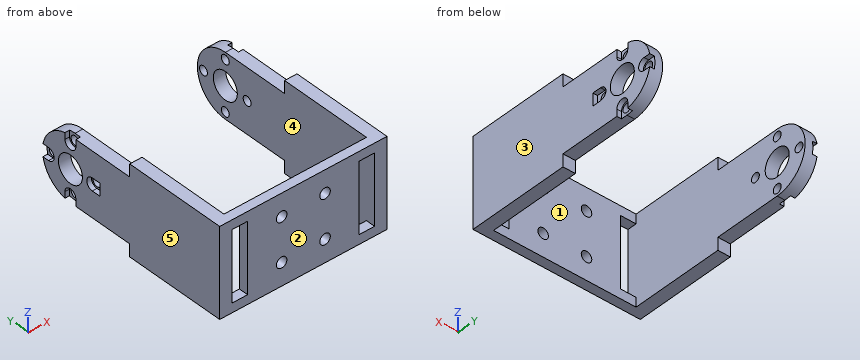
```python
from build123d import *
from build123d.topology import SkipClean

# Parameters (mm, degrees)
SKETCH1_W           = 54
SKETCH1_H           = 28.5
SKETCH1_W_2         = 5
SKETCH1_H_2         = 22.5
SKETCH1_R           = 1.7
SKETCH1_R_2         = 7.5
BOSS_EXTRUDE2_DEPTH = 3
SKETCH2_W           = 4
SKETCH2_H           = 20.5
BOSS_EXTRUDE3_DEPTH = 21.75
SKETCH4_R           = 10.25
BOSS_EXTRUDE4_DEPTH = 4
SKETCH6_R           = 4.4
SKETCH6_R_2         = 1.45
CUT_EXTRUDE3_DEPTH  = 4
SKETCH7_R           = 1.45
CUT_EXTRUDE4_DEPTH  = 1.5
SKETCH8_W           = 28.781481152
SKETCH8_H           = 28.5
BOSS_EXTRUDE5_DEPTH = 3
SKETCH9_R           = 1.7
CUT_EXTRUDE5_DEPTH  = 3
SKETCH10_W          = 54
SKETCH10_H          = 28.5
SKETCH10_R          = 1.7
SKETCH10_W_2        = 5
SKETCH10_H_2        = 22.5
BOSS_EXTRUDE7_DEPTH = 30
SKETCH11_W          = 46
SKETCH11_H          = 30
CUT_EXTRUDE6_DEPTH  = 30


with BuildPart() as part:
    # Sketch1 → Boss-Extrude2 (new body)
    with BuildSketch(Plane(origin=(0, 0, 0), x_dir=(1, 0, 0), z_dir=(0, 1, 0))):
        Rectangle(SKETCH1_W, SKETCH1_H)
        with Locations((20.5, 0)):
            Rectangle(SKETCH1_W_2, SKETCH1_H_2, mode=Mode.SUBTRACT)
        with Locations((-20.5, 0)):
            Rectangle(SKETCH1_W_2, SKETCH1_H_2, mode=Mode.SUBTRACT)
        with Locations(Location((-9, -8.25, 0), (0, 0, 270))):
            Circle(SKETCH1_R, mode=Mode.SUBTRACT)
        with Locations(Location((9, -8.25, 0), (0, 0, 270))):
            Circle(SKETCH1_R, mode=Mode.SUBTRACT)
        with Locations(Location((-9, 8.25, 0), (0, 0, 270))):
            Circle(SKETCH1_R, mode=Mode.SUBTRACT)
        with Locations(Location((0, 0, 0), (0, 0, 270))):
            Circle(SKETCH1_R_2, mode=Mode.SUBTRACT)
        with Locations(Location((9, 8.25, 0), (0, 0, 270))):
            Circle(SKETCH1_R, mode=Mode.SUBTRACT)
    extrude(amount=BOSS_EXTRUDE2_DEPTH)

    # Sketch2 → Boss-Extrude3 (add)
    with BuildSketch(Plane(origin=(0, 3, 0), x_dir=(1, 0, 0), z_dir=(0, 1, 0))):
        with Locations((25, 0)):
            Rectangle(SKETCH2_W, SKETCH2_H)
    boss_extrude3 = extrude(amount=BOSS_EXTRUDE3_DEPTH)

    # Sketch4 → Boss-Extrude4 (add)
    with BuildSketch(Plane(origin=(27, 0, 0), x_dir=(0, 0, -1), z_dir=(1, 0, 0))):
        with Locations((0, 24.75)):
            Circle(SKETCH4_R)
    boss_extrude4 = extrude(amount=-BOSS_EXTRUDE4_DEPTH)

    # Mirror1: Boss-Extrude3, Boss-Extrude4 across plane
    add(boss_extrude3.mirror(Plane(origin=(0, 0, 0), x_dir=(0, 0, 1), z_dir=(1, 0, 0))))
    add(boss_extrude4.mirror(Plane(origin=(0, 0, 0), x_dir=(0, 0, 1), z_dir=(1, 0, 0))))

    # Sketch6 → Cut-Extrude3 (cut)
    with BuildSketch(Plane(origin=(27, 0, 0), x_dir=(0, 0, -1), z_dir=(1, 0, 0))):
        with Locations((0, 24.75)):
            Circle(SKETCH6_R)
        with Locations((0, 32.75)):
            Circle(SKETCH6_R_2)
        with Locations((8, 24.75)):
            Circle(SKETCH6_R_2)
        with Locations((0, 16.75)):
            Circle(SKETCH6_R_2)
        with Locations((-8, 24.75)):
            Circle(SKETCH6_R_2)
    cut_extrude3 = extrude(amount=-CUT_EXTRUDE3_DEPTH, mode=Mode.SUBTRACT)

    # Mirror3: Cut-Extrude3 across plane
    add(cut_extrude3.mirror(Plane(origin=(0, 0, 0), x_dir=(0, 0, 1), z_dir=(1, 0, 0))), mode=Mode.SUBTRACT)

    # Sketch7 → Cut-Extrude4 (cut)
    # profile 1 of 4: a face of its own
    with BuildSketch(Plane(origin=(27, 0, 0), x_dir=(0, 0, -1), z_dir=(1, 0, 0))):
        with BuildLine():
            ThreePointArc((10.25, 24.75), (10.200627247, 25.754840168), (10.052984631, 26.75))
            Line((10.052984631, 26.75), (8, 26.75))
            ThreePointArc((8, 26.75), (6, 24.75), (8, 22.75))
            Line((8, 22.75), (10.25, 22.75))
            Line((10.25, 22.75), (10.25, 24.75))
        make_face()
        with Locations((8, 24.75)):
            Circle(SKETCH7_R, mode=Mode.SUBTRACT)
    # profile 2 of 4: a face of its own
    with BuildSketch(Plane(origin=(27, 0, 0), x_dir=(0, 0, -1), z_dir=(1, 0, 0))):
        with BuildLine():
            Line((2, 32.75), (2, 34.802984631))
            ThreePointArc((2, 34.802984631), (0, 35), (-2, 34.802984631))
            Line((-2, 34.802984631), (-2, 32.75))
            ThreePointArc((-2, 32.75), (0, 30.75), (2, 32.75))
        make_face()
        with Locations((0, 32.75)):
            Circle(SKETCH7_R, mode=Mode.SUBTRACT)
    # profile 3 of 4: a face of its own
    with BuildSketch(Plane(origin=(27, 0, 0), x_dir=(0, 0, -1), z_dir=(1, 0, 0))):
        with BuildLine():
            Line((-8, 26.75), (-10.052984631, 26.75))
            ThreePointArc((-10.052984631, 26.75), (-10.200627247, 25.754840168), (-10.25, 24.75))
            Line((-10.25, 24.75), (-10.25, 22.75))
            Line((-10.25, 22.75), (-8, 22.75))
            ThreePointArc((-8, 22.75), (-6, 24.75), (-8, 26.75))
        make_face()
        with Locations((-8, 24.75)):
            Circle(SKETCH7_R, mode=Mode.SUBTRACT)
    # profile 4 of 4: a face of its own
    with BuildSketch(Plane(origin=(27, 0, 0), x_dir=(0, 0, -1), z_dir=(1, 0, 0))):
        with BuildLine():
            Line((-2, 16.75), (-2, 13.927640071))
            Line((-2, 13.927640071), (2, 13.927640071))
            Line((2, 13.927640071), (2, 16.75))
            ThreePointArc((2, 16.75), (0, 18.75), (-2, 16.75))
        make_face()
        with Locations((0, 16.75)):
            Circle(SKETCH7_R, mode=Mode.SUBTRACT)
    cut_extrude4 = extrude(amount=-CUT_EXTRUDE4_DEPTH, mode=Mode.SUBTRACT)

    # Mirror4: Cut-Extrude4 across plane
    add(cut_extrude4.mirror(Plane(origin=(0, 0, 0), x_dir=(0, 0, 1), z_dir=(1, 0, 0))), mode=Mode.SUBTRACT)

    # Sketch8 → Boss-Extrude5 (add)
    with BuildSketch(Plane(origin=(0, 3, 0), x_dir=(1, 0, 0), z_dir=(0, 1, 0))):
        Rectangle(SKETCH8_W, SKETCH8_H)
    extrude(amount=-BOSS_EXTRUDE5_DEPTH)

    # Sketch9 → Cut-Extrude5 (cut)
    with BuildSketch(Plane(origin=(0, 3, 0), x_dir=(1, 0, 0), z_dir=(0, 1, 0))):
        with BuildLine():
            ThreePointArc((-5.3, -7), (-5.797918472, -5.797918472), (-7, -5.3))
            Line((-7, -5.3), (-7, -7))
            Line((-7, -7), (-5.3, -7))
        make_face()
        with BuildLine():
            Line((-7, -7), (-7, -5.3))
            ThreePointArc((-7, -5.3), (-8.202081528, -8.202081528), (-5.3, -7))
            Line((-5.3, -7), (-7, -7))
        make_face()
        with BuildLine():
            ThreePointArc((8.7, -7), (8.202081528, -5.797918472), (7, -5.3))
            Line((7, -5.3), (7, -7))
            Line((7, -7), (5.3, -7))
            ThreePointArc((5.3, -7), (7, -8.7), (8.7, -7))
        make_face()
        with BuildLine():
            Line((7, -7), (7, -5.3))
            ThreePointArc((7, -5.3), (5.797918472, -5.797918472), (5.3, -7))
            Line((5.3, -7), (7, -7))
        make_face()
        with BuildLine():
            ThreePointArc((8.7, 7), (7, 8.7), (5.3, 7))
            Line((5.3, 7), (7, 7))
            Line((7, 7), (7, 5.3))
            ThreePointArc((7, 5.3), (8.202081528, 5.797918472), (8.7, 7))
        make_face()
        with BuildLine():
            Line((7, 7), (5.3, 7))
            ThreePointArc((5.3, 7), (5.797918472, 5.797918472), (7, 5.3))
            Line((7, 5.3), (7, 7))
        make_face()
        with Locations(Location((-7, 7, 0), (0, 0, 270))):
            Circle(SKETCH9_R)
    extrude(amount=-CUT_EXTRUDE5_DEPTH, mode=Mode.SUBTRACT)

    # Sketch10 → Boss-Extrude7 (add)
    with SkipClean():  # the faces are left unmerged after this step: merging them gives an invalid solid
        with BuildSketch(Plane.XZ):
            Rectangle(SKETCH10_W, SKETCH10_H)
            with Locations(Location((-7, 7, 0), (0, 0, 90))):
                Circle(SKETCH10_R, mode=Mode.SUBTRACT)
            with Locations(Location((7, 7, 0), (0, 0, 90))):
                Circle(SKETCH10_R, mode=Mode.SUBTRACT)
            with Locations(Location((7, -7, 0), (0, 0, 90))):
                Circle(SKETCH10_R, mode=Mode.SUBTRACT)
            with Locations(Location((-7, -7, 0), (0, 0, 90))):
                Circle(SKETCH10_R, mode=Mode.SUBTRACT)
            with Locations((-20.5, 0)):
                Rectangle(SKETCH10_W_2, SKETCH10_H_2, mode=Mode.SUBTRACT)
            with Locations((20.5, 0)):
                Rectangle(SKETCH10_W_2, SKETCH10_H_2, mode=Mode.SUBTRACT)
        extrude(amount=BOSS_EXTRUDE7_DEPTH)

    # Sketch11 → Cut-Extrude6 (cut)
    with BuildSketch(Plane.XY.offset(14.25)):
        with Locations((0, -12)):
            Rectangle(SKETCH11_W, SKETCH11_H)
    extrude(amount=-CUT_EXTRUDE6_DEPTH, mode=Mode.SUBTRACT)


solid = part.part
```
Work out the finished part from the listing and answer in its coordinate system (mm). Face numbers are marked on the shaded views. A direction names the side the tool comes from. Give positions to 0.01 mm unless a question says otherwise; leave off trailing zeros. Write each loop counter-clockwise with the first axis right and the second up, starting at its lowest first coordinate (ties: lowest second). Pieces come first, ordered by that corner, then holes.
(1) The part is cut by section C-C on z = 0. Count the separate pieces of the cut face and the enclosed holes in it, plus the area to 3 significant figures.
Final values:
separate pieces: 9
enclosed holes: 0
area: 501 mm2
(2) The mould has two halves that part along X. Classify the marked faces 3, 4 and 5: pulls with the +X half, pulls with the -X half, needs draft (parallel to the pull), parting line crosses it, or undercut.
Final values:
face 3: pulls with the +X half
face 4: undercut
face 5: pulls with the -X half
(3) The part is cut by section B-B on x = -22. Write down the section's boundary in (y, z), plus the area to 3 significant figures.
Final values:
outline: (-30, -14.25) - (-27, -14.25) - (-27, -11.25) - (-30, -11.25) - close; (-30, 11.25) - (-27, 11.25) - (-27, 14.25) - (-30, 14.25) - close
area: 18.0 mm2
(4) Straight lines are drawn through the part: line 1 (Y direction, x = -24.25, z = 0); line 2 (X direction, y = -27.8, z = -7); line 3 (X direction, y = -20.5, z = 8.5). For each, find the intervals that lie inside material, in ascending order.
Final values:
line 1: y = -30 to 15.3, 18.2 to 20.35, 29.15 to 31.3, 34.2 to 35
line 2: x = -27 to -23, -18 to -8.7, -5.3 to 5.3, 8.7 to 18, 23 to 27
line 3: x = -27 to -23, 23 to 27
(5) Flat-ended cylindrical pins translate along their axes: pin 1 Ø5.5 at (x, z) = (7, 7) entering from +Y; pin 2 Ø1.6 at (x, y) = (26, 15.5) entering from +Z; pin 3 Ø5 at (x, y) = (20, -8) entering from -Z; pin 4 Ø1.2 at (y, z) = (17.5, 0.5) entering from -X. Find the tip coordinate at first contact, or state that the pin passes through.
Final values:
pin 1: stops at y = -27
pin 2: stops at z = 10.25
pin 3: passes through
pin 4: stops at x = -25.5
(6) The part is cut by section D-D on x = 0.5. Write down the section's boundary in (y, z).
Final values:
outline: (-30, -14.25) - (-27, -14.25) - (-27, 14.25) - (-30, 14.25) - close
(7) Which of the six approach directions +Z, -Z, +X, -X, +Y, -Y give full straight-line access (tool end or side, diameter ignored) to the marked faces 1 and 2?
Final values:
face 1: +Z, -Z, +Y
face 2: +Z, -Z, +X, -X, -Y
(8) The part is cut by section A-A on y = 12.5. Write down the section's boundary in (x, z).
Final values:
outline: (-27, -10.25) - (-23, -10.25) - (-23, 10.25) - (-27, 10.25) - close; (23, -10.25) - (27, -10.25) - (27, 10.25) - (23, 10.25) - close
